CAD build for the part. Positions are in the model's coordinates, mm. Face numbers are marked on the shaded views. A direction names the side the tool comes from. Give positions to 0.01 mm unless a question says otherwise; leave off trailing zeros. Loops run counter-clockwise (first coordinate to the right, second up) from the corner with the lowest first, then second, coordinate; pieces in that order, holes last. Notation, with made-up numbers: (39, -32.5) - (51, -32.5) arc R25 cw to (51, -8.5) - close; hole circle Ø3 at (31, 82). An arc over 180 degrees is marked (long way). Return JSON: item names as keys, results as strings.
from build123d import *

# Parameters (mm, degrees)
SKETCH1_R                = 5
BOSS_EXTRUDE1_DEPTH      = 30
SKETCH3_R                = 5
BOSS_EXTRUDE2_DEPTH      = 10
BOSS_EXTRUDE2_DEPTH_BACK = 10
SKETCH5_R                = 2.5
BOSS_EXTRUDE3_DEPTH      = 5
BOSS_EXTRUDE3_DEPTH_BACK = 25
SKETCH6_R                = 2.5
BOSS_EXTRUDE4_DEPTH      = 5
BOSS_EXTRUDE4_DEPTH_BACK = 35


with BuildPart() as part:
    # Sketch1 → Boss-Extrude1 (new body)
    with BuildSketch(Plane.XY):
        Circle(SKETCH1_R)
    extrude(amount=-BOSS_EXTRUDE1_DEPTH)

    # Sketch3 → Boss-Extrude2 (add, two sides)
    with BuildSketch(Plane(origin=(0, 0, 0), x_dir=(0, 0, -1), z_dir=(1, 0, 0))) as boss_extrude2_sk:
        with Locations((15, 0)):
            Circle(SKETCH3_R)
    extrude(amount=BOSS_EXTRUDE2_DEPTH)
    extrude(boss_extrude2_sk.sketch, amount=-BOSS_EXTRUDE2_DEPTH_BACK)

    # Sketch5 → Boss-Extrude3 (add, two sides)
    with BuildSketch(Plane(origin=(10, 0, 0), x_dir=(0, 0, -1), z_dir=(1, 0, 0))) as boss_extrude3_sk:
        with Locations((15, 0)):
            Circle(SKETCH5_R)
    extrude(amount=BOSS_EXTRUDE3_DEPTH)
    extrude(boss_extrude3_sk.sketch, amount=-BOSS_EXTRUDE3_DEPTH_BACK)

    # Sketch6 → Boss-Extrude4 (add, two sides)
    with BuildSketch(Plane.XY) as boss_extrude4_sk:
        Circle(SKETCH6_R)
    extrude(amount=BOSS_EXTRUDE4_DEPTH)
    extrude(boss_extrude4_sk.sketch, amount=-BOSS_EXTRUDE4_DEPTH_BACK)


solid = part.part
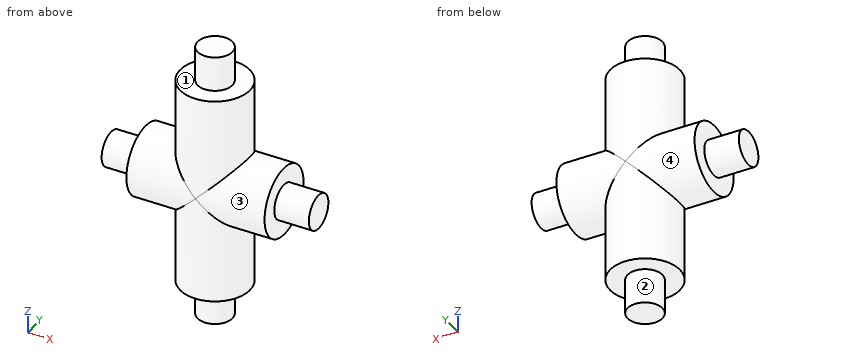
1. Drop flat-ended pins along their axis: P1, Ø3, axis at x = 7, y = -3, coming from the -Z side; P2, Ø12, axis at x = 10.5, z = -30.5, coming from the -Y side; P3, Ø4, axis at y = -0.5, z = -26, coming from the -X side. Give the stop position or say it passes through.
Values follow:
{"P1": "stops at z = -19.77", "P2": "stops at y = -2.14", "P3": "stops at x = -5"}
2. Cut at B-B, the plane z = -22. Write the cut outline in (x, y), plus the area to 3 significant figures.
Values follow:
{"outline": "circle Ø10 at (0, 0)", "area": "78.5 mm²"}
3. Cut at A-A, the plane y = 0. Write the cut outline in (x, z), plus the area to 3 significant figures.
Values follow:
{"outline": "(-15, -17.5) - (-10, -17.5) - (-10, -20) - (-5, -20) - (-5, -30) - (-2.5, -30) - (-2.5, -35) - (2.5, -35) - (2.5, -30) - (5, -30) - (5, -20) - (10, -20) - (10, -17.5) - (15, -17.5) - (15, -12.5) - (10, -12.5) - (10, -10) - (5, -10) - (5, 0) - (2.5, 0) - (2.5, 5) - (-2.5, 5) - (-2.5, 0) - (-5, 0) - (-5, -10) - (-10, -10) - (-10, -12.5) - (-15, -12.5) - close", "area": "500 mm²"}
4. Cut at C-C, the plane x = 6.25. Write the cut outline in (y, z).
Values follow:
{"outline": "circle Ø10 at (0, -15)"}
5. Cut at D-D, the plane y = 4.25. Write the cut outline in (x, z).
Values follow:
{"outline": "(-10, -17.63) - (-2.63, -17.63) - (-2.63, -30) - (2.63, -30) - (2.63, -17.63) - (10, -17.63) - (10, -12.37) - (2.63, -12.37) - (2.63, 0) - (-2.63, 0) - (-2.63, -12.37) - (-10, -12.37) - close"}
6. Drill centre lines: probe 1 along Z at (x, y) = (-3.25, -0.75); probe 2 along X at (y, z) = (-0.5, -10.5); probe 3 along Z at (x, y) = (8.75, 1.5). Where is each one in solid material? Low to high.
Values follow:
{"probe 1": "z = -30 to 0", "probe 2": "x = -10 to 10", "probe 3": "z = -19.77 to -10.23"}
7. Which spindle directions (+Z, -Z, +X, -X, +Y, -Y) get a long thin tool onto all of the face, cutting with end or side? Do the marked faces 1, 2, 3 and 4. Say none if no direction does.
Values follow:
{"face 1": "+Z", "face 2": "-Z", "face 3": "+X", "face 4": "-X"}
